Build history of the part. All positions in model axes, mm. A direction names the side the tool comes from. Round coordinates to 2 decimals unless told otherwise and drop trailing zeros. Order: outer loops, then holes, each group sorted by start corner. A loop starts at its lowest first (then second) coordinate and runs counter-clockwise, first axis right, second up. Notation, with made-up numbers: M -29,85 L 20,85 A12 ccw 20,97 Z; hole C 56.5,46.5 d2. An arc over 180 degrees is marked long. One line per item, written item: value. Start each with the question number.
Item 1: Band-saw the part on B-B, the plane x = 0. Write the cut outline in (y, z) (3 decimals), then the cut area to 3 significant figures.
Item 2: Pin check, flat tips, straight feed: pin 1 (4.5 mm diameter, centred on x = 0, y = 8.509, fed in from +Z); pin 2 (6 mm diameter, centred on x = 3.5, y = 9.5, fed in from -Z); pin 3 (3.5 mm diameter, centred on x = 0, y = 8.5, fed in from +Z). Stop position of each tip, or through.
Item 3: Two-plate mould, pull along X, no slides. Class faces 1 (the cylindrical face through (-2.637, 8.454, -11.877)), 2 (the cylindrical face through (-0.562, 2.318, 26.342)), 3 (the flat face through (5.2, 12.446, -0.2)), 4 (the cylindrical face through (-0.562, 2.318, -21.283)): +X half, -X half, draft (parallel to the pull), parting line (faces both ways), or undercut.
Item 4: Band-saw the part on A-A, the plane z = 0. Write the cut outline in (x, y) (3 decimals).
Item 5: Band-saw the part on D-D, the plane y = 11.5. Write the cut outline in (x, z).
Item 6: Probe L1, parallel to Z at x = 0, y = 3.3 (3 decimals); L2, parallel to Z at x = 21.5, y = 2.5; L3, parallel to Z at x = -1, y = 1.25. List the from-to ranges inside material, lowest first.
Item 7: Band-saw the part on C-C, the plane x = -20. Write the cut outline in (y, z).
Item 8: Tool access for faces 5 (the cylindrical face through (-0.44, 6.54, 8.02)), 6 (the flat face through (0, 0, -6)), 7 (the flat face through (0, 6, -3.753)), 8 (the flat face through (-12, 4.572, -6)): list every direction of +Z, -Z, +X, -X, +Y, -Y with a clear straight run to the whole face (end or side of a thin tool).
Autodesk Inventor part; units mm, degrees
ref_plane "YZ Plane" through (0, 0, 0) normal (1, 0, 0) x (0, 1, 0)
ref_plane "XZ Plane" through (0, 0, 0) normal (0, 1, 0) x (-1, 0, 0)
ref_plane "XY Plane" through (0, 0, 0) normal (0, 0, 1) x (1, 0, 0)
sketch "Sketch1" plane through (0, 0, 0) normal (0, 1, 0) x (-1, 0, 0)
  circle A0 centre (0, 0) radius 28.575
  dimension "d0" = 57.15
extrude "Extrusion1" add sketch "Sketch1" along normal blind 4.572
sketch "Sketch2" plane through (0, 4.572, 0) normal (0, 1, 0) x (1, 0, 0)
  circle A0 centre (0, 0) radius 28.575
  circle A1 centre (0, 0) radius 12.1666
  dimension "d3" = 24.3332
extrude "Extrusion2" add sketch "Sketch2" along normal blind 7.874 contours A1
sketch "Sketch3" plane through (0, 4.572, 0) normal (0, 1, 0) x (1, 0, 0)
  circle A0 centre (0, 0) radius 28.575
  circle A1 centre (0, 0) radius 23.8125 construction
  circle A2 centre (0, 23.8125) radius 2.5908
  line L0 (0, 0) -> (0, 23.8125) construction
  circle A3 centre (-20.6222, 11.9063) radius 2.5908
  circle A4 centre (-20.6222, -11.9062) radius 2.5908
  circle A5 centre (0, -23.8125) radius 2.5908
  circle A6 centre (20.6222, -11.9063) radius 2.5908
  circle A7 centre (20.6222, 11.9062) radius 2.5908
  dimension "d6" = 47.625
  dimension "d7" = 5.1816
  dimension "d10" = 360
extrude "Extrusion3" cut sketch "Sketch3" against normal blind 7.874 contours A2 | A3 | A4 | A5 | A6 | A7
sketch "Sketch4" plane through (0, 12.446, 0) normal (0, 1, 0) x (1, 0, 0)
  circle A0 centre (0, 0) radius 12.1666
  line L0 (-3.304, 3.7529) -> (3.304, 3.7529)
  line L1 (-3.304, -3.7528) -> (3.304, -3.7528)
  line L2 (3.304, 3.7529) -> (3.304, -3.7528) construction
  line L3 (-3.304, 3.7529) -> (-3.304, -3.7528) construction
  arc A1 (-3.304, 3.7529) -> (-3.304, -3.7528) centre (0, 0) ccw
  arc A2 (3.304, -3.7528) -> (3.304, 3.7529) centre (0, 0) ccw
  dimension "d15" = 7.5057
  dimension "d16" = 5
  dimension "d17" = 5
extrude "Extrusion4" cut sketch "Sketch4" against normal blind 14.986 contours L0 A2 L1 A1
ref_plane "Work Plane1" through (0, 4.572, 12.1666) normal (0, 0, 1) x (1, 0, 0)
sketch "Sketch5" plane through (0, 4.572, 12.1666) normal (0, 0, 1) x (1, 0, 0)
  circle A0 centre (0, 3.937) radius 2.0193
  line L0 (0, -4.572) -> (0, 3.937) construction
  line L1 (-28.575, -4.572) -> (28.575, -4.572) construction
  dimension "d20" = 8.509
  dimension "d21" = 4.0386
extrude "Extrusion5" cut sketch "Sketch5" against normal blind 12.3698
properties part number "Snowblower Hub"
Output:
1. outline: M 0,-28.575 L 4.572,-28.575 L 4.572,-26.403 L 0,-26.403 Z; M 0,-21.222 L 4.572,-21.222 L 4.572,-12.167 L 12.446,-12.167 L 12.446,-3.753 L 0,-3.753 Z; M 0,3.753 L 6.49,3.753 L 6.49,12.167 L 4.572,12.167 L 4.572,21.222 L 0,21.222 Z; M 0,26.403 L 4.572,26.403 L 4.572,28.575 L 0,28.575 Z; M 10.528,3.753 L 12.446,3.753 L 12.446,12.167 L 10.528,12.167 Z
1. area: 278 mm²
2. pin 1: stops at z = 12.17
2. pin 2: stops at z = -12.16
2. pin 3: stops at z = -3.75
3. face 1: parting line
3. face 2: undercut
3. face 3: draft
3. face 4: undercut
4. outline: M -28.575,0 L -5,0 L -5,12.446 L -12.167,12.446 L -12.167,4.572 L -28.575,4.572 Z; M 5,0 L 28.575,0 L 28.575,4.572 L 12.167,4.572 L 12.167,12.446 L 5,12.446 Z
5. outline: C 0,0 d24.33; hole M -3.3,-3.75 L 3.3,-3.75 A5 ccw 3.3,3.75 L -3.3,3.75 A5 ccw Z
6. L1: z = -28.575 to -26.403, -21.222 to -3.753, 3.753 to 21.222, 26.403 to 28.575
6. L2: z = -18.82 to -14.34, -9.47 to 9.47, 14.34 to 18.82
6. L3: z = -28.56 to -26.2, -21.42 to -3.75, 3.75 to 21.42, 26.2 to 28.56
7. outline: M 0,-20.41 L 4.57,-20.41 L 4.57,-14.42 L 0,-14.42 Z; M 0,-9.39 L 4.57,-9.39 L 4.57,9.39 L 0,9.39 Z; M 0,14.42 L 4.57,14.42 L 4.57,20.41 L 0,20.41 Z
8. face 5: +Z
8. face 6: +Z, -Z, +X, -X, -Y
8. face 7: +Y, -Y
8. face 8: +Y
